Geometry: final body of the model. Coordinates: model frame, mm. A direction names the side the tool comes from. Coordinates: 2 decimals unless noted, no trailing zeros. Order: outer loops, then holes, each group sorted by start corner. A loop starts at its lowest first (then second) coordinate and runs counter-clockwise, first axis right, second up. Notation, with made-up numbers: M 9.25,23 L 20.25,23 A13 ccw 20.25,28 Z; hole C -8,4 d8. An arc over 180 degrees is marked long. Use CSV: the item, a comma, the result in double quotes. Start each with the question number.
Q1. Ray query, probe 1 along Z at (x, y) = (0.6, 0.75); probe 2 along Y at (x, z) = (1.7, -17.5); probe 3 along Y at (x, z) = (1.55, -42.5). Return the intervals inside material, ascending.
Q2. Section query D-D, the plane z = -8. Output: boundary loops of the cut face in (x, y), and give its area (3 significant figures).
Q3. Access query for faces 5 (the face through (1, -1, -29)), 6 (the face through (1, 0.5, -31.5)), 7 (the face through (1, -1, -32)), 8 (the face through (1, 2.6, -6)). Directions: +Z, -Z, +X, -X, +Y, -Y. A direction counts if a zero-diameter tool reaches every point of the face in a straight line with its end or side. Return the directions, or none.
Q4. Section query C-C, the plane z = -24. Output: boundary loops of the cut face in (x, y).
Q5. Section query B-B, the plane x = 1.45. Output: boundary loops of the cut face in (y, z).
Q6. Section query A-A, the plane y = 0.5. Output: boundary loops of the cut face in (x, z).
Q7. Mould query, pull axis Y, two halves, no side actions, for faces 1 (the face through (1, 1.5, -46)), 2 (the face through (1.014, 2.756, -11.947)), 3 (the face through (1, -0.5, -46)), 4 (the face through (1, 1, 0)). Classes: +Y half, -Y half, draft (parallel to the pull), parting line (faces both ways), or undercut.
Q8. First-contact query: P1, Ø1.2, axis at x = 1, y = -0.5, coming from the -Z side; P2, Ø0.6, axis at x = 0.5, z = -45.5, coming from the -Y side; P3, Ø0.6, axis at x = 0.5, z = -3.5, coming from the +Y side. Flat tips, straight axial feed; report the tip coordinate or a pass-through.
from build123d import *

# Parameters (mm, degrees)
SKETCH_1_W      = 12
SKETCH_1_H      = 2.6
EXTRUDE_1_DEPTH = 2
FILLET_1_R      = 2


with BuildPart() as part:
    # Эскиз1 → Бобышка-Вытянуть1 (new body)
    with BuildSketch(Plane(origin=(0, 0, 0), x_dir=(0, 0, -1), z_dir=(1, 0, 0))):
        Polygon((48, 1), (48, 4.6), (29, 4.6), (14, 4.6), (12, 2.6), (12, 0), (29, 0), (29, -1.5), (32, -1.5), (32, 0), (31, 1), (31, 2), (46, 2), (46, 1), (45, 0), (45, -0.5), (47, -0.5), (47, 0), align=None)
        with Locations((6, 1.3)):
            Rectangle(SKETCH_1_W, SKETCH_1_H)
    extrude(amount=EXTRUDE_1_DEPTH)

    # Скругление1
    fillet_1_edges = [part.edges().sort_by_distance(p)[0] for p in [
        (1, 2.6, -12),
        (1, 4.6, -14),
    ]]
    fillet(fillet_1_edges, radius=FILLET_1_R)


solid = part.part
Responses:
1,probe 1,"z = -47.75 to -45.75, -31.25 to 0"
1,probe 2,"y = 0 to 4.6"
1,probe 3,"y = 2 to 4.6"
2,outline,"M 0,0 L 2,0 L 2,2.6 L 0,2.6 Z"
2,area,"5.20 mm²"
3,face 5,"+Z, +X, -X, -Y"
3,face 6,"+X, -X"
3,face 7,"+X, -X, -Y"
3,face 8,"+Z, +X, -X, +Y"
4,outline,"M 0,0 L 2,0 L 2,4.6 L 0,4.6 Z"
5,outline,"M -1.5,-32 L 0,-32 L 1,-31 L 2,-31 L 2,-46 L 1,-46 L 0,-45 L -0.5,-45 L -0.5,-47 L 0,-47 L 1,-48 L 4.6,-48 L 4.6,-14.83 A2 ccw 4.01,-13.41 L 3.19,-12.59 A2 cw 2.6,-11.17 L 2.6,0 L 0,0 L 0,-29 L -1.5,-29 Z"
6,outline,"M 0,-47.5 L 2,-47.5 L 2,-45.5 L 0,-45.5 Z; M 0,-31.5 L 2,-31.5 L 2,0 L 0,0 Z"
7,face 1,"undercut"
7,face 2,"+Y half"
7,face 3,"-Y half"
7,face 4,"draft"
8,P1,"stops at z = -47.1"
8,P2,"stops at y = -0.5"
8,P3,"stops at y = 2.6"
